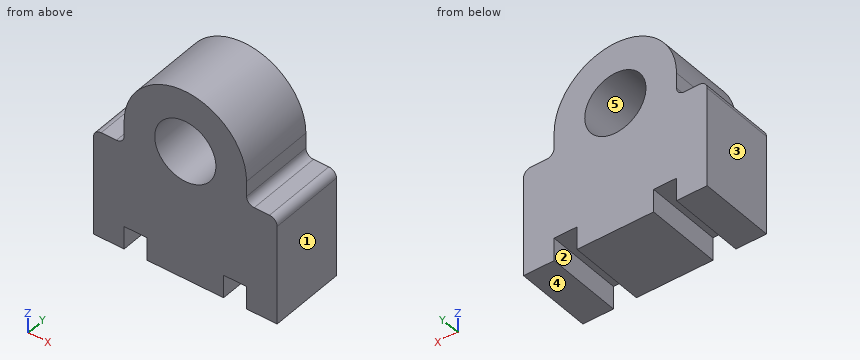
Autodesk Fusion 360 part; units mm, degrees
sketch "Sketch1" plane through (0, 0, 0) normal (0, 1, 0) x (1, 0, 0)
  line L0 (-147.5, 45) -> (-147.5, -95)
  line L1 (92.5, -95) -> (92.5, 45)
  line L2 (52.5, 45) -> (52.5, 15)
  line L3 (22.5, 15) -> (22.5, 45)
  line L4 (52.5, 15) -> (22.5, 15)
  line L5 (-107.5, 45) -> (-107.5, 15)
  line L6 (-107.5, 15) -> (-77.5, 15)
  line L7 (-77.5, 15) -> (-77.5, 45)
  line L8 (-107.5, 45) -> (-147.5, 45)
  line L9 (92.5, 45) -> (52.5, 45)
  line L10 (22.5, 45) -> (-77.5, 45)
  line L11 (-107.5, -95) -> (-107.5, -125)
  line L12 (52.5, -125) -> (52.5, -95)
  line L13 (-147.5, -95) -> (-107.5, -95)
  line L14 (52.5, -95) -> (92.5, -95)
  arc A0 (-107.5, -125) -> (52.5, -125) centre (-27.5, -125) ccw
  dimension "d1" = 40
  dimension "d2" = 30
  dimension "d3" = 40
  dimension "d4" = 30
  dimension "d5" = 100
  dimension "d6" = 30
  dimension "d7" = 30
  dimension "d8" = 120
  dimension "d9" = 140
  dimension "d10" = 40
  dimension "d11" = 170
extrude "Extrude1" add sketch "Sketch1" along normal blind 100
sketch "Sketch2" plane through (0, 0, 0) normal (0, -1, 0) x (1, 0, 0)
  line L0 (-147.5, -45) -> (-107.5, -45)
  line L1 (-107.5, -45) -> (-107.5, -15)
  line L2 (-107.5, -15) -> (-77.5, -15)
  line L3 (-77.5, -15) -> (-77.5, -45)
  line L4 (-77.5, -45) -> (22.5, -45)
  line L5 (22.5, -45) -> (22.5, -15)
  line L6 (22.5, -15) -> (52.5, -15)
  line L7 (52.5, -15) -> (52.5, -45)
  line L8 (52.5, -45) -> (92.5, -45)
  line L9 (92.5, -45) -> (92.5, 95)
  line L10 (92.5, 95) -> (52.5, 95)
  line L11 (52.5, 95) -> (52.5, 125)
  arc A0 (52.5, 125) -> (-107.5, 125) centre (-27.5, 125) ccw
  line L12 (-107.5, 125) -> (-107.5, 95)
  line L13 (-107.5, 95) -> (-147.5, 95)
  line L14 (-147.5, 95) -> (-147.5, -45)
  circle A1 centre (-27.5, 125) radius 40
  dimension "d14" = 80
extrude "Extrude2" cut sketch "Sketch2" against normal blind 100 contours A1
fillet "Fillet1" radius 10 2 edges at (52.5, 50, 95) (-107.5, 50, 95)
fillet "Fillet2" radius 10 2 edges at (92.5, 50, 95) (-147.5, 50, 95)
Work out the finished part from the listing and answer in its coordinate system (mm). Face numbers are marked on the shaded views. A direction names the side the tool comes from. Give positions to 0.01 mm unless a question says otherwise; leave off trailing zeros. Loops run counter-clockwise (first coordinate to the right, second up) from the corner with the lowest first, then second, coordinate; pieces in that order, holes last. Notation, with made-up numbers: (11.25, 61.5) - (64.25, 61.5) arc R35 cw to (64.25, 93.5) - close; hole circle Ø7 at (-37, -13). An arc over 180 degrees is marked (long way). Use CSV: the item, a comma, the result in double quotes. Start each with the question number.
(1) Find section A-A, the plane x = -27.5. Determine the outline of the cut face in (y, z), plus the area to 3 significant figures.
(2) Find the intervals of material crossed by L1, parallel to X at y = 64.5, z = -22.5; L2, parallel to Z at x = -27.5, y = 40; L3, parallel to X at y = 30, z = 98.5, in increasing order.
(3) Each of these flat-tipped pins is pushed along its axis until it touches: pin 1 (22 mm diameter, centred on x = -131.5, y = 67.5, fed in from +Z); pin 2 (10 mm diameter, centred on x = 9, z = 114, fed in from +Y); pin 3 (9 mm diameter, centred on x = -85.5, y = 27, fed in from -Z); pin 4 (12 mm diameter, centred on y = 67.5, z = 137, fed in from -X). Where does it stop, or does it pass through?
(4) Find section B-B, the plane y = 8.5. Determine the outline of the cut face in (x, z).
(5) Determine the mould class of the marked faces 3, 4 and 5 for opening direction X: released by +X, released by -X, zero draft, split by the parting line, or undercut.
(6) Find section C-C, the plane x = -86.5. Determine the outline of the cut face in (y, z).
(7) A tool of negligible diameter and unlimited length cuts with its end or side. For the marked faces 1 and 2, from which of +Z, -Z, +X, -X, +Y, -Y can it reach the whole face along a straight path? Write none if from no direction.
Results found:
1,outline,"(0, -45) - (100, -45) - (100, 85) - (0, 85) - close; (0, 165) - (100, 165) - (100, 205) - (0, 205) - close"
1,area,"17,000 mm^2"
2,L1,"-147.5 to -107.5, -77.5 to 22.5, 52.5 to 92.5"
2,L2,"-45 to 85, 165 to 205"
2,L3,"-109.9 to -57.46, 2.46 to 54.9"
3,pin 1,"z = 95"
3,pin 2,"y = 100"
3,pin 3,"z = -15"
3,pin 4,"x = -107.27"
4,outline,"(-147.5, -45) - (-107.5, -45) - (-107.5, -15) - (-77.5, -15) - (-77.5, -45) - (22.5, -45) - (22.5, -15) - (52.5, -15) - (52.5, -45) - (92.5, -45) - (92.5, 85) arc R10 ccw to (82.5, 95) - (62.5, 95) arc R10 cw to (52.5, 105) - (52.5, 125) arc R80 ccw to (-107.5, 125) - (-107.5, 105) arc R10 cw to (-117.5, 95) - (-137.5, 95) arc R10 ccw to (-147.5, 85) - close; hole circle Ø80 at (-27.5, 125)"
5,face 3,"released by -X"
5,face 4,"zero draft"
5,face 5,"undercut"
6,outline,"(0, -15) - (100, -15) - (100, 179.03) - (0, 179.03) - close"
7,face 1,"+Z, -Z, +X, +Y, -Y"
7,face 2,"-Z, +Y, -Y"
